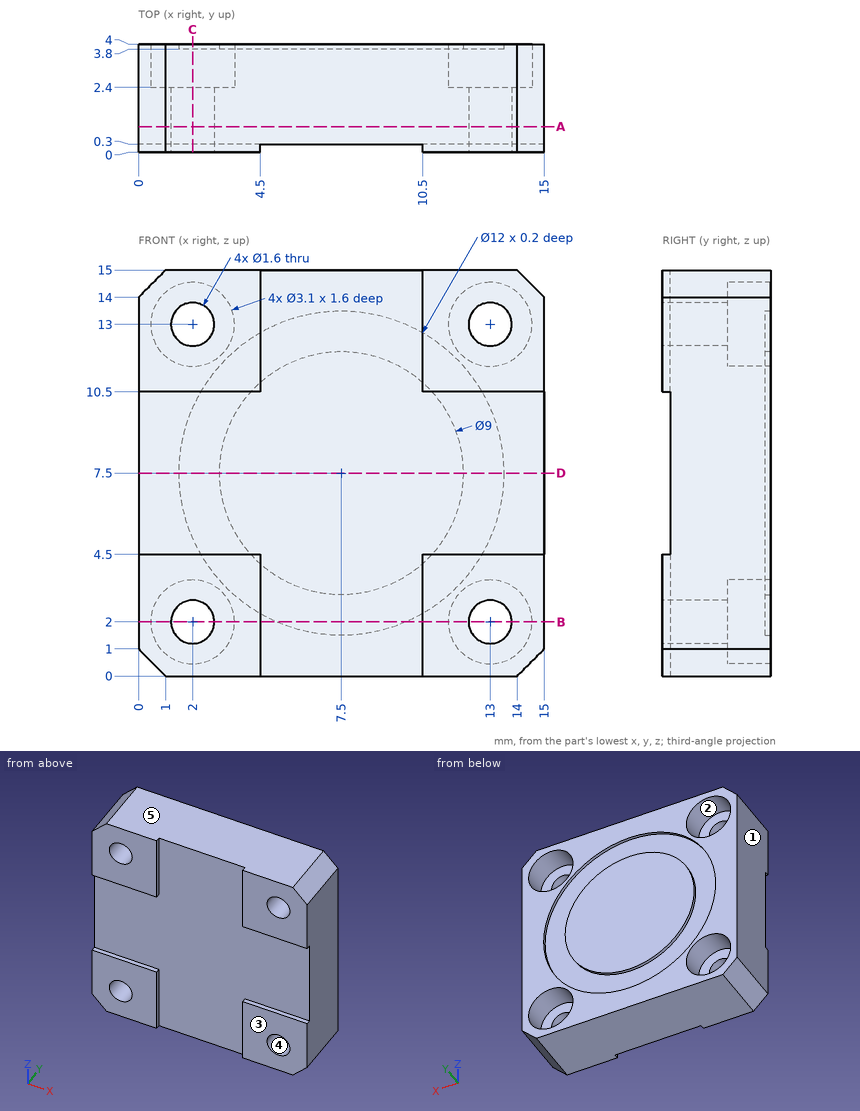
The figure shows three views and two pictorial views of one solid part (mm, origin at its lowest corner). Answer the questions. A direction names the side the tool comes from. Round coordinates to 2 decimals unless told otherwise and drop trailing zeros. Write each loop counter-clockwise with the first axis right and the second up, starting at its lowest first coordinate (ties: lowest second). Pieces come first, ordered by that corner, then holes. Notation, with made-up numbers: (11, 40) - (35, 40) arc R31 cw to (35, 75) - close; hole circle Ø11 at (-1, 50.5). An arc over 180 degrees is marked (long way). Answer in a Markdown table with one row per item. Add a question column.
1. The mould has two halves that part along Z. Classify the marked faces 3, 4 and 5: +Z half, -Z half, draft (parallel to the pull), parting line (faces both ways), or undercut.
2. A cutting plane is placed at B-B, the plane z = 2. Determine the outline of the cut face in (x, y).
3. A cutting plane is placed at C-C, the plane x = 2. Determine the outline of the cut face in (y, z), and give its area (3 significant figures).
4. Find the intervals of material crossed by line 1 along Z through (x, y) = (13, 1); line 2 along Z through (x, y) = (7.5, 3.95); line 3 along X through (y, z) = (3.45, 2), in increasing order. Write a range as from..to.
5. For the marked faces 1 and 2, determine the directions among +Z, -Z, +X, -X, +Y, -Y from which every point of the face is accessible in a straight line to the end or side of a thin tool.
6. A cutting plane is placed at A-A, the plane y = 0.95. Determine the outline of the cut face in (x, z).
7. Given pin 1 (1 mm diameter, centred on x = 2, z = 2, fed in from +Y); pin 2 (0.9 mm diameter, centred on x = 1.5, z = 2.5, fed in from +Y); pin 3 (1 mm diameter, centred on x = 8, z = 10.5, fed in from -Y), each flat-ended and moving along its own axis, determine where each tip first touches the part or whether it passes through.
8. A cutting plane is placed at D-D, the plane z = 7.5. Determine the outline of the cut face in (x, y), and give its area (3 significant figures).
Worked out:
| question | item | result |
|---|---|---|
| 1 | face 3 | draft |
| 1 | face 4 | undercut |
| 1 | face 5 | +Z half |
| 2 | outline | (0, 0) - (1.2, 0) - (1.2, 2.4) - (0.45, 2.4) - (0.45, 4) - (0, 4) - close; (2.8, 0) - (4.5, 0) - (4.5, 0.3) - (10.5, 0.3) - (10.5, 0) - (12.2, 0) - (12.2, 2.4) - (11.45, 2.4) - (11.45, 4) - (9.9, 4) - (9.9, 3.8) - (5.1, 3.8) - (5.1, 4) - (3.55, 4) - (3.55, 2.4) - (2.8, 2.4) - close; (13.8, 0) - (15, 0) - (15, 4) - (14.55, 4) - (14.55, 2.4) - (13.8, 2.4) - close |
| 3 | outline | (0, 0) - (4, 0) - (4, 0.45) - (2.4, 0.45) - (2.4, 1.2) - (0, 1.2) - close; (0, 2.8) - (2.4, 2.8) - (2.4, 3.55) - (4, 3.55) - (4, 5.1) - (3.8, 5.1) - (3.8, 9.9) - (4, 9.9) - (4, 11.45) - (2.4, 11.45) - (2.4, 12.2) - (0, 12.2) - (0, 10.5) - (0.3, 10.5) - (0.3, 4.5) - (0, 4.5) - close; (0, 13.8) - (2.4, 13.8) - (2.4, 14.55) - (4, 14.55) - (4, 15) - (0, 15) - close |
| 3 | area | 39.6 mm^2 |
| 4 | line 1 | 0..1.2, 2.8..12.2, 13.8..15 |
| 4 | line 2 | 0..1.5, 3..12, 13.5..15 |
| 4 | line 3 | 0..0.45, 3.55..11.45, 14.55..15 |
| 5 | face 1 | +Z, -Z, -X, +Y, -Y |
| 5 | face 2 | +Y |
| 6 | outline | (0, 1) - (1, 0) - (14, 0) - (15, 1) - (15, 14) - (14, 15) - (1, 15) - (0, 14) - close; hole circle Ø1.6 at (2, 2); hole circle Ø1.6 at (2, 13); hole circle Ø1.6 at (13, 2); hole circle Ø1.6 at (13, 13) |
| 7 | pin 1 | through |
| 7 | pin 2 | y = 2.4 |
| 7 | pin 3 | y = 0.3 |
| 8 | outline | (0, 0.3) - (15, 0.3) - (15, 4) - (13.5, 4) - (13.5, 3.8) - (12, 3.8) - (12, 4) - (3, 4) - (3, 3.8) - (1.5, 3.8) - (1.5, 4) - (0, 4) - close |
| 8 | area | 54.9 mm^2 |
